The listing builds one solid part. Answer for the finished solid, in the listing's coordinates (mm). A direction names the side the tool comes from. Round coordinates to 2 decimals unless told otherwise and drop trailing zeros. Loops run counter-clockwise (first coordinate to the right, second up) from the corner with the lowest first, then second, coordinate; pieces in that order, holes last. Notation, with made-up numbers: (57.5, 38) -> (108.5, 38) arc R15 ccw to (108.5, 49) -> close; hole circle Ø2 at (86, 48). An arc over 180 degrees is marked (long way). Use a Markdown table: item, result. Add a question column.
Q1. Given pin 1 Ø1.8 at (y, z) = (-77, 2) entering from -X; pin 2 Ø1.5 at (x, y) = (6, -52) entering from +Z; pin 3 Ø1.3 at (y, z) = (-31.5, 4.5) entering from -X; pin 4 Ø8 at (x, y) = (4, -48) entering from -Z, each flat-ended and moving along its own axis, determine where each tip first touches the part or whether it passes through.
Q2. Which of the six approach directions +Z, -Z, +X, -X, +Y, -Y give full straight-line access (tool end or side, diameter ignored) to faces 1 (the flat face through (2.96, -20.29, 1.77)), 2 (the flat face through (0, -37, 2)), 3 (the flat face through (7, -49, 3.6))?
Q3. Section D-D on x = 7.5 is taken. Give the vertices of the cut face in (y, z).
Q4. Section A-A on x = 2 is taken. Give the vertices of the cut face in (y, z) (1 decimal), then the cut area to 3 significant figures.
Q5. Section B-B on y = -26 is taken. Give the vertices of the cut face in (x, z).
Q6. For a pull along Y with two mould halves and no side action, classify faces 4 (the flat face through (7, 0, 1)), 5 (the flat face through (2.958, -30.861, 1.825)), 6 (the flat face through (9, -49, 0)) as released by +Y, released by -Y, zero draft, split by the parting line, or undercut.
Q7. Section C-C on z = 1.95 is taken. Give the vertices of the cut face in (x, y) (3 decimals).
Q8. Consider line 1 (Y direction, x = 2, z = 2.35); line 2 (Z direction, x = 1, y = -62); line 3 (Y direction, x = 3, z = 2.65). Determine where each line is inside the solid, lowest interval first.
from build123d import *

# Parameters (mm, degrees)
BASE_DEPTH   = 99.2
JOIN_1_DEPTH = 6
CROQUIS3_W   = 9.6
CROQUIS3_H   = 99.2
JOIN_2_DEPTH = 0.4


with BuildPart() as part:
    # Croquis1 → BASE (new body)
    with BuildSketch(Plane(origin=(0, 0, 0), x_dir=(-1, 0, 0), z_dir=(0, 1, 0))):
        Polygon((0, 0), (-18.6, 0), (-9.6, 5.2), (-9.6, 4), (0, 4), align=None)
    extrude(amount=-BASE_DEPTH)

    # Croquis2 → JOIN_1 (cut)
    with BuildSketch(Plane(origin=(0, 0, 0), x_dir=(0, -1, 0), z_dir=(-1, 0, 0))):
        Polygon((18.35, -0.4), (21.925, 3.6), (29.275, 3.6), (32.85, -0.4), align=None)
        Polygon((40.85, -0.4), (44.425, 3.6), (54.775, 3.6), (58.35, -0.4), align=None)
        Polygon((69.925, 3.6), (66.35, -0.4), (80.85, -0.4), (77.275, 3.6), align=None)
    extrude(amount=-JOIN_1_DEPTH, mode=Mode.SUBTRACT)

    # Croquis3 → JOIN_2 (cut)
    with BuildSketch(Plane.XY.offset(4)):
        with Locations((4.8, -49.6)):
            Rectangle(CROQUIS3_W, CROQUIS3_H)
    extrude(amount=-JOIN_2_DEPTH, mode=Mode.SUBTRACT)


solid = part.part
Checked values:
| question | item | result |
|---|---|---|
| 1 | pin 1 | stops at x = 6 |
| 1 | pin 2 | stops at z = 3.6 |
| 1 | pin 3 | stops at x = 9.6 |
| 1 | pin 4 | stops at z = 0 |
| 2 | face 1 | -Z, -X |
| 2 | face 2 | +Z, -Z, -X, +Y, -Y |
| 2 | face 3 | +Z, -X, +Y, -Y |
| 3 | outline | (-99.2, 0) -> (0, 0) -> (0, 3.6) -> (-99.2, 3.6) -> close |
| 4 | outline | (-99.2, 0) -> (-80.5, 0) -> (-77.3, 3.6) -> (-99.2, 3.6) -> close; (-69.9, 3.6) -> (-66.7, 0) -> (-58, 0) -> (-54.8, 3.6) -> close; (-44.4, 3.6) -> (-41.2, 0) -> (-32.5, 0) -> (-29.3, 3.6) -> close; (-21.9, 3.6) -> (-18.7, 0) -> (0, 0) -> (0, 3.6) -> close |
| 4 | area | 232 mm2 |
| 5 | outline | (6, 0) -> (18.6, 0) -> (9.6, 5.2) -> (9.6, 3.6) -> (6, 3.6) -> close |
| 6 | face 4 | released by +Y |
| 6 | face 5 | undercut |
| 6 | face 6 | zero draft |
| 7 | outline | (0, -99.2) -> (15.225, -99.2) -> (15.225, 0) -> (0, 0) -> (0, -20.45) -> (6, -20.45) -> (6, -30.75) -> (0, -30.75) -> (0, -42.95) -> (6, -42.95) -> (6, -56.25) -> (0, -56.25) -> (0, -68.45) -> (6, -68.45) -> (6, -78.75) -> (0, -78.75) -> close |
| 8 | line 1 | y = -99.2 to -78.39, -68.81 to -55.89, -43.31 to -30.39, -20.81 to 0 |
| 8 | line 2 | z = 0 to 3.6 |
| 8 | line 3 | y = -99.2 to -78.12, -69.08 to -55.62, -43.58 to -30.12, -21.08 to 0 |
